from build123d import *

# Parameters (mm, degrees)
F0_R     = 28.575
F0_R_2   = 7.9375
F1_DEPTH = 12.7
F2_W     = 3.175
F2_H     = 6.35
F5_R     = 1.5875
F6_DEPTH = 25.4


with BuildPart() as f1:
    # F0 (on Front) → F1 (new body)
    with BuildSketch(Plane.XZ):
        Circle(F0_R)
        with Locations((9.525, 0)):
            Circle(F0_R_2, mode=Mode.SUBTRACT)
    extrude(amount=F1_DEPTH)

    # F2 (on Top) → F4 (revolve, cut)
    with BuildSketch(Plane.XY):
        with Locations((26.9875, -6.35)):
            Rectangle(F2_W, F2_H)
    revolve(axis=Axis((-0.004353, -5.31878, 0), (0.000473, -1, 0)), mode=Mode.SUBTRACT)

    # F5 (on Right) → F6 (cut)
    with BuildSketch(Plane.YZ):
        with Locations((-6.35, 0)):
            Circle(F5_R)
    extrude(amount=F6_DEPTH, mode=Mode.SUBTRACT)


solid = f1.part
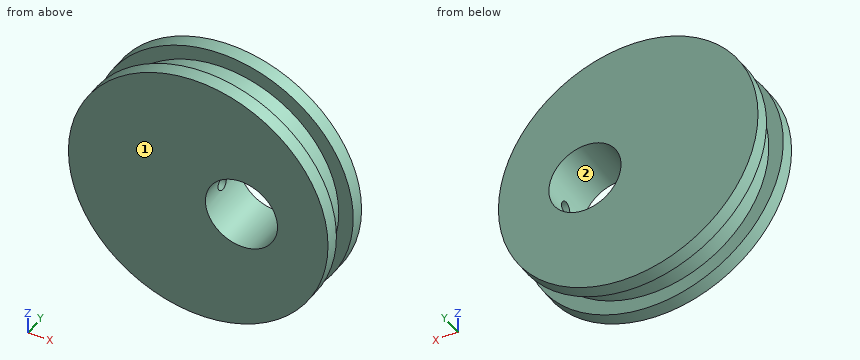
Input: part model. Units: mm. Frame: model coordinates. Face numbers are marked on the shaded views. Coordinates: 2 decimals unless noted, no trailing zeros. Answer in a Markdown table with one row per item.
(1) Section query B-B, the plane z = 0. Give the number of separate pieces and of enclosed holes in the cut face, plus the area to 3 significant figures.
Numbers:
| item | result |
|---|---|
| separate pieces | 3 |
| enclosed holes | 0 |
| area | 454 mm^2 |
(2) Draft query along Z for the marked faces 1 and 2. Return one class per face: pulls with the +Z half, pulls with the -Z half, needs draft (parallel to the pull), parting line crosses it, or undercut.
Numbers:
| item | result |
|---|---|
| face 1 | needs draft |
| face 2 | undercut |
(3) Contact query for flat-ended pins moving along their axis: pin 1 Ø3.5 at (y, z) = (-6.35, 0) entering from +X; pin 2 Ø6 at (y, z) = (-9, 1) entering from -X (3 decimals); pin 3 Ø3 at (x, y) = (-12.5, -7.5) entering from -Z; pin 4 Ø1.5 at (x, y) = (-3.5, -8.5) entering from +Z. Output: stop coordinate, or through.
Numbers:
| item | result |
|---|---|
| pin 1 | stops at x = 25.4 |
| pin 2 | stops at x = -28.575 |
| pin 3 | stops at z = -22.9 |
| pin 4 | stops at z = 25.25 |
(4) Material intervals for line 1 (Y direction, x = 20, z = -17); line 2 (X direction, y = -2.75, z = 0) (1 decimal); line 3 (Y direction, x = 24, z = 0), sorted ascending. Write a range as [from, to].
Numbers:
| item | result |
|---|---|
| line 1 | y = [-12.7, -9.53], [-3.18, 0] |
| line 2 | x = [-28.6, 1.6], [17.5, 28.6] |
| line 3 | y = [-12.7, -7.94], [-4.76, 0] |
